Here's how the part is built. I have some questions about the finished solid (model axes, mm). Coordinates: 2 decimals unless noted, no trailing zeros. Write each loop counter-clockwise with the first axis right and the second up, starting at its lowest first coordinate (ties: lowest second). Pieces come first, ordered by that corner, then holes.
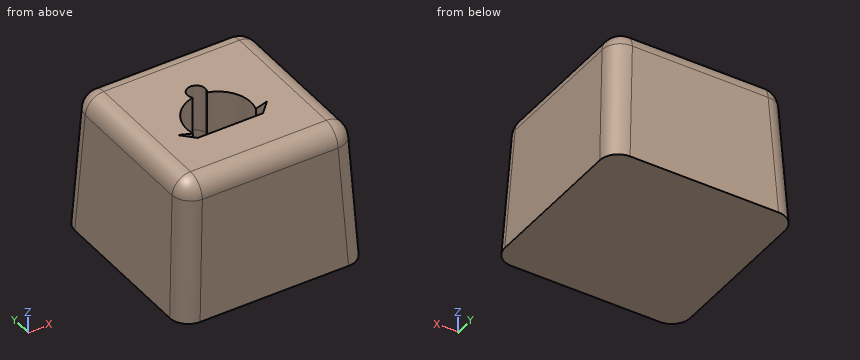
from build123d import *

# Parameters (mm, degrees)
F0_W     = 20
F0_H     = 20
F1_DEPTH = 15
F1_TAPER = 3
F2_R     = 2
F4_DEPTH = 5
F6_DEPTH = 2


with BuildPart() as f1:
    # F0 (on Top) → F1 (new body)
    with BuildSketch(Plane.XY):
        with Locations((1.9706902094, 0.2862163961)):
            Rectangle(F0_W, F0_H)
    extrude(amount=F1_DEPTH, taper=F1_TAPER)

    # F2
    f2_edges = [f1.edges().sort_by_distance(p)[0] for p in [
        (11.577632, 9.893158, 7.5),
        (1.97069, 9.5001, 15),
        (-7.636251, 9.893158, 7.5),
        (11.184574, 0.286216, 15),
        (11.577632, -9.320725, 7.5),
        (1.97069, -8.927667, 15),
        (-7.243193, 0.286216, 15),
        (-7.636251, -9.320725, 7.5),
    ]]
    fillet(f2_edges, radius=F2_R)

    # F3 (on face) → F4 (cut)
    with BuildSketch(Plane.XY.offset(15)):
        with BuildLine():
            ThreePointArc((2.4668298597, 2.420319631), (2.6270550618, 2.7065444383), (2.6825853886, 3.0298293568))
            ThreePointArc((2.6825853886, 3.0298293568), (1.4060278584, 3.9484621473), (0.9404779675, 2.446214288))
            ThreePointArc((0.9404779675, 2.446214288), (1.6973410612, 2.0611579891), (2.4668298597, 2.420319631))
        make_face()
        with BuildLine():
            ThreePointArc((2.4668298597, 2.420319631), (1.6973410612, 2.0611579891), (0.9404779675, 2.446214288))
            ThreePointArc((0.9404779675, 2.446214288), (-1.5061031251, 0.7291430041), (-2.005701419, -2.2178036161))
            Line((-2.005701419, -2.2178036161), (-3.3031930216, -1.6699736007))
            Line((-3.3031930216, -1.6699736007), (-2.005701419, -3.0136309616))
            Line((-2.005701419, -3.0136309616), (5.0295870751, -3.0136309616))
            Line((5.0295870751, -3.0136309616), (6.3270786777, -1.6699736007))
            Line((6.3270786777, -1.6699736007), (4.8565878533, -2.0736376755))
            ThreePointArc((4.8565878533, -2.0736376755), (4.6201459688, 0.6830104281), (2.4668298597, 2.420319631))
        make_face()
    extrude(amount=-F4_DEPTH, mode=Mode.SUBTRACT)

    # F5 (on face) → F6 (cut)
    with BuildSketch(Plane.XY.offset(10)):
        with BuildLine():
            ThreePointArc((0.9404779675, 2.446214288), (-0.7753137079, 1.5817313603), (-1.8659088252, 0))
            ThreePointArc((-1.8659088252, 0), (-1.0221589161, -0.6510962238), (0, -0.3493822005))
            ThreePointArc((0, -0.3493822005), (0.6882312009, -0.8328877124), (1.3764624018, -0.3493822005))
            ThreePointArc((1.3764624018, -0.3493822005), (1.9947274122, -0.8549416092), (2.6129924227, -0.3493822005))
            ThreePointArc((2.6129924227, -0.3493822005), (3.1948891701, -0.6762140192), (3.7767859176, -0.3493822005))
            ThreePointArc((3.7767859176, -0.3493822005), (4.4330516654, -0.4840787766), (4.8961884025, 0))
            ThreePointArc((4.8961884025, 0), (3.9955688533, 1.5253924233), (2.4668298597, 2.420319631))
            ThreePointArc((2.4668298597, 2.420319631), (1.7302082041, 3.9985007245), (0.9404779675, 2.446214288))
        make_face()
    extrude(amount=-F6_DEPTH, mode=Mode.SUBTRACT)


solid = f1.part
1. I want a section at B-B (x = -4.5). List the corners of the cut face in (y, z) for me, then the cut area to 3 significant figures.
2. If I drill on line 1 (Y direction, x = 1.75, z = 10.5); line 2 (X direction, y = 3.5, z = 10); line 3 (X direction, y = 3.75, z = 12), over which ranges is the centre line in solid material (lowest first)?
3. I want a section at A-A (y = 4.5). List the corners of the cut face in (x, z) for me, then the cut area to 3 significant figures.
4. For pin 1 Ø2.5 at (x, y) = (1, 1) entering from +Z; pin 2 Ø5.5 at (x, z) = (2, 11.5) entering from +Y; pin 3 Ø6 at (x, z) = (5, 4.5) entering from -Y; pin 4 Ø3 at (x, y) = (1.71, 3.03) entering from +Z, each with a flat end and sliding along its axis, tell me the tip position at first contact or that it passes through.
5. I want a section at C-C (x = -0.5). List the corners of the cut face in (y, z) for me.
Response values:
1. outline: (-9.71, 0) - (10.29, 0) - (9.6, 13.1) arc R2 ccw to (7.6, 15) - (-7.03, 15) arc R2 ccw to (-9.03, 13.1) - close
1. area: 287 mm2
2. line 1: y = -9.16 to -3.01, 4 to 9.74
2. line 2: x = -7.51 to 0.87, 2.56 to 11.45
2. line 3: x = -7.4 to 1.07, 2.36 to 11.34
3. outline: (-8.03, 0) - (11.97, 0) - (11.28, 13.1) arc R2 ccw to (9.29, 15) - (-5.35, 15) arc R2 ccw to (-7.34, 13.1) - close
3. area: 287 mm2
4. pin 1: stops at z = 8
4. pin 2: stops at y = 9.83
4. pin 3: stops at y = -9.64
4. pin 4: stops at z = 15
5. outline: (-9.71, 0) - (10.29, 0) - (9.6, 13.1) arc R2 ccw to (7.6, 15) - (1.8, 15) - (1.8, 8) - (-0.63, 8) - (-0.63, 10) - (-3.01, 10) - (-3.01, 15) - (-7.03, 15) arc R2 ccw to (-9.03, 13.1) - close
